from build123d import *

# Parameters (mm, degrees)
F0_W     = 4
F0_H     = 7.471158
F0_W_2   = 2
F0_H_2   = 4
F0_H_3   = 6.5
F2_SIZE2 = 0.5
F2_SIZE  = 0.5


with BuildPart() as f1:
    # F0 (on Front) → F1 (revolve)
    with BuildSketch(Plane.XZ):
        with Locations((-2, 11.264421)):
            Rectangle(F0_W, F0_H)
        Polygon((0, 5.75), (0, 7.528842), (-4, 7.528842), (-3.75, 5.75), align=None)
        Polygon((0, 4), (0, 5.75), (-3.75, 5.75), (-2, 4), align=None)
        with Locations((-1, 2)):
            Rectangle(F0_W_2, F0_H_2)
        Polygon((0, -2), (0, 0), (-2, 0), (-4, -2), align=None)
        with Locations((-2, -5.25)):
            Rectangle(F0_W, F0_H_3)
        with BuildLine():
            Line((0, -12.5), (0, -8.5))
            Line((0, -8.5), (-4, -8.5))
            ThreePointArc((-4, -8.5), (-2.828427, -11.328427), (0, -12.5))
        make_face()
    revolve(axis=Axis((0, 0, 1.25), (0, 0, -1)))

    # F2
    f2_edges = [f1.edges().sort_by_distance(p)[0] for p in [
        (4, 0, 15),
    ]]
    chamfer(f2_edges, length=F2_SIZE, length2=F2_SIZE2)


solid = f1.part
Work out the finished part from the listing and answer in its coordinate system (mm). A direction names the side the tool comes from. Give positions to 0.01 mm unless a question says otherwise; leave off trailing zeros. Loops run counter-clockwise (first coordinate to the right, second up) from the corner with the lowest first, then second, coordinate; pieces in that order, holes last. Notation, with made-up numbers: (24, 84) -> (42, 84) arc R31 ccw to (42, 122) -> close; hole circle Ø2 at (30.25, 7). An arc over 180 degrees is marked (long way). Use a Markdown table: item, result. Add a question column.
1. Section A-A on z = 2.5 is taken. Determine the outline of the cut face in (x, y), and give its area (3 significant figures).
2. Determine the mould class of faces 1 (the conical face through (3.008, -2.306, 6.034)), 2 (the cylindrical face through (0.867, -3.905, 11.063)), 3 (the flat face through (0, 0, 15)) for opening direction Z: released by +Z, released by -Z, zero draft, split by the parting line, or undercut.
3. Flat-ended cylindrical pins translate along their axes: pin 1 Ø2 at (x, z) = (-0.5, -7) entering from -Y; pin 2 Ø1.5 at (x, z) = (-2, 7.5) entering from +Y; pin 3 Ø3 at (x, z) = (2.5, 4) entering from -Y. Find the tip coordinate at first contact, or state that the pin passes through.
4. Find the intervals of material crossed by probe 1 along Z at (x, y) = (2.75, -0.25); probe 2 along Z at (x, y) = (2.5, 1.5); probe 3 along X at (y, z) = (3.5, 12), in increasing order.
5. Section B-B on z = 10.75 is taken. Determine the outline of the cut face in (x, y), and give its area (3 significant figures).
6. For faces 4 (the cylindrical face through (0, -2, 2)), 5 (the cylindrical face through (0.867, -3.905, -5.204)), determine the directions among +Z, -Z, +X, -X, +Y, -Y from which every point of the face is accessible in a straight line to the end or side of a thin tool.
Results below:
| question | item | result |
|---|---|---|
| 1 | outline | circle Ø4 at (0, 0) |
| 1 | area | 12.6 mm^2 |
| 2 | face 1 | undercut |
| 2 | face 2 | zero draft |
| 2 | face 3 | released by +Z |
| 3 | pin 1 | stops at y = -4 |
| 3 | pin 2 | stops at y = 3.8 |
| 3 | pin 3 | stops at y = -2.8 |
| 4 | probe 1 | z = -11.39 to -0.76, 4.76 to 15 |
| 4 | probe 2 | z = -11.24 to -0.92, 4.92 to 15 |
| 4 | probe 3 | x = -1.94 to 1.94 |
| 5 | outline | circle Ø8 at (0, 0) |
| 5 | area | 50.3 mm^2 |
| 6 | face 4 | none |
| 6 | face 5 | +Z, -Z |
